```python
from build123d import *

# Parameters (mm, degrees)
F0_W     = 47.024399
F0_H     = 54.634411
F1_DEPTH = 25.4
F2_W     = 20.959661
F2_H     = 10.561608
F3_DEPTH = 50.8
F4_R     = 4.569204
F5_DEPTH = 42.271631


with BuildPart() as f1:
    # F0 (on Front) → F1 (new body)
    with BuildSketch(Plane.XZ):
        with Locations((23.512199, 27.317206)):
            Rectangle(F0_W, F0_H)
    extrude(amount=F1_DEPTH)

    # F2 (on face) → F3 (join)
    with BuildSketch(Plane(origin=(0, 0, 0), x_dir=(-1, 0, 0), z_dir=(0, 1, 0))):
        with Locations((-23.303836, 36.989827)):
            Rectangle(F2_W, F2_H)
        with Locations((-21.026581, 17.570276)):
            Rectangle(F2_W, F2_H)
    extrude(amount=F3_DEPTH)

    # F4 (on face) → F5 (cut, through all)
    with BuildSketch(Plane.XY.offset(42.270631)):
        with Locations((21.938689, 30.440513)):
            Circle(F4_R)
    extrude(amount=-F5_DEPTH, mode=Mode.SUBTRACT)


solid = f1.part
```
Source: CAD feature listing. Evaluate the final solid. Frame: model axes, mm. A direction names the side the tool comes from. Coordinates: 2 decimals unless noted, no trailing zeros. Loops run counter-clockwise (first coordinate to the right, second up) from the corner with the lowest first, then second, coordinate; pieces in that order, holes last. Notation, with made-up numbers: (-32.75, 6.5) -> (0.25, 6.5) arc R19 cw to (0.25, 26.5) -> close; hole circle Ø11 at (25.25, 68.25). An arc over 180 degrees is marked (long way). One line per item, written item: value. Start each with the question number.
Q1. Section query A-A, the plane y = 8.5. Return the cut outline in (x, z), and give its area (3 significant figures).
Q2. Mould query, pull axis Y, two halves, no side actions, for faces 6 (the face through (24.05, 26.39, 37.06)), 7 (the face through (24.05, 26.39, 17.64)), 8 (the face through (21, 50.8, 18)), 9 (the face through (21, 25, 12.289)). Classes: pulls with the +Y half, pulls with the -Y half, needs draft (parallel to the pull), parting line crosses it, or undercut.
Q3. Section query D-D, the plane x = 19. Return the cut outline in (y, z), and give its area (3 significant figures).
Q4. Section query B-B, the plane x = 29. Return the cut outline in (y, z), and give its area (3 significant figures).
Q5. Section query C-C, the plane z = 40. Return the cut outline in (x, y).
Q6. Line query: line 1 along Z through (x, y) = (23.5, 46); line 2 along Y through (x, z) = (37, 21); line 3 along X through (y, z) = (11.5, 20). Output: solid intervals per line, ascending.
Q7. Set-up query: faces 1 (the face through (10.547, 25, 17)), 2 (the face through (12.824, 25, 37)), 3 (the face through (31.506, 25, 17)), 4 (the face through (21, 25, 22.851)), 5 (the face through (33.784, 25, 37)). Return all of +Z, -Z, +X, -X, +Y, -Y with unobstructed straight access to the full face (end or side cutting, diameter ignored); none if empty.
Q8. Contact query for flat-ended pins moving along their axis: P1, Ø11.5, axis at y = 30, z = 15.5, coming from the +X side; P2, Ø5.5, axis at y = 30.5, z = 34.5, coming from the -X side; P3, Ø1, axis at y = 17, z = 12, coming from the -X side; P4, Ø8, axis at x = 21.94, y = 30.44, coming from the +Z side. Output: stop coordinate, or through.
Results:
1. outline: (10.55, 12.29) -> (31.51, 12.29) -> (31.51, 22.85) -> (10.55, 22.85) -> close; (12.82, 31.71) -> (33.78, 31.71) -> (33.78, 42.27) -> (12.82, 42.27) -> close
1. area: 443 mm^2
2. face 6: undercut
2. face 7: undercut
2. face 8: pulls with the +Y half
2. face 9: needs draft
3. outline: (-25.4, 0) -> (0, 0) -> (0, 12.29) -> (26.94, 12.29) -> (26.94, 22.85) -> (0, 22.85) -> (0, 31.71) -> (26.94, 31.71) -> (26.94, 42.27) -> (0, 42.27) -> (0, 54.63) -> (-25.4, 54.63) -> close; (33.94, 12.29) -> (50.8, 12.29) -> (50.8, 22.85) -> (33.94, 22.85) -> close; (33.94, 31.71) -> (50.8, 31.71) -> (50.8, 42.27) -> (33.94, 42.27) -> close
3. area: 2,310 mm^2
4. outline: (-25.4, 0) -> (0, 0) -> (0, 12.29) -> (50.8, 12.29) -> (50.8, 22.85) -> (0, 22.85) -> (0, 31.71) -> (50.8, 31.71) -> (50.8, 42.27) -> (0, 42.27) -> (0, 54.63) -> (-25.4, 54.63) -> close
4. area: 2,460 mm^2
5. outline: (0, -25.4) -> (47.02, -25.4) -> (47.02, 0) -> (33.78, 0) -> (33.78, 50.8) -> (12.82, 50.8) -> (12.82, 0) -> (0, 0) -> close; hole circle Ø9.14 at (21.94, 30.44)
6. line 1: 12.29 to 22.85, 31.71 to 42.27
6. line 2: -25.4 to 0
6. line 3: 10.55 to 31.51
7. face 1: +Z, -Z, -X, +Y
7. face 2: +Z, -X, +Y
7. face 3: -Z, +X, +Y
7. face 4: +X, -X, +Y
7. face 5: +Z, -Z, +X, +Y
8. P1: x = 31.51
8. P2: x = 12.82
8. P3: x = 10.55
8. P4: through
